Geometry check sheet. Reference: the model listing, model coordinates, mm. Face numbers are marked on the shaded views. A direction names the side the tool comes from. Give positions to 0.01 mm unless a question says otherwise; leave off trailing zeros. Order: outer loops, then holes, each group sorted by start corner. A loop starts at its lowest first (then second) coordinate and runs counter-clockwise, first axis right, second up. Notation, with made-up numbers: M -12,57.25 L 20,57.25 A37 ccw 20,94.25 Z; hole C -34.5,-9 d4. An arc over 180 degrees is marked long. Answer as a JSON object with one key per item and string values. Group by question number.
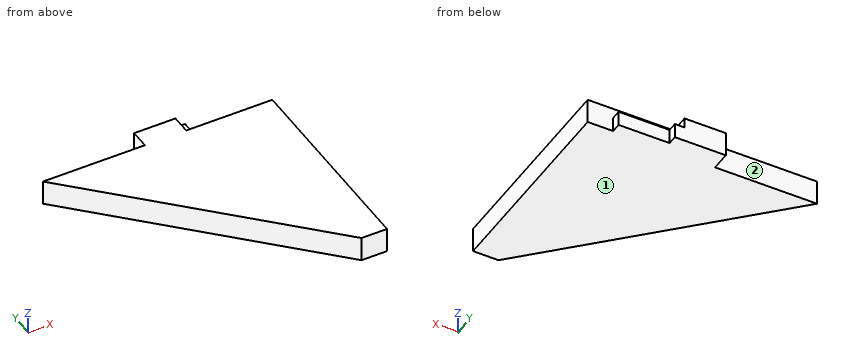
from build123d import *

# Parameters (mm, degrees)
F0_W     = 10.287
F0_H     = 4.745708
F0_W_2   = 6.35
F0_H_2   = 50.8
F1_DEPTH = 6.223
F0_W_3   = 12.7
F0_H_3   = 2.413
F2_DEPTH = 3.683


with BuildPart() as f1:
    # F0 (on Top) → F1 (new body)
    with BuildSketch(Plane.XY):
        Polygon((-25.4, 25.4), (25.4, -25.4), (25.4, 25.4), (12.7, 25.4), (10.287, 25.4), (0, 25.4), align=None)
        with Locations((5.1435, 27.772854)):
            Rectangle(F0_W, F0_H)
        with Locations((28.575, 0)):
            Rectangle(F0_W_2, F0_H_2)
    extrude(amount=F1_DEPTH)

    # F0 (on Top) → F2 (join)
    with BuildSketch(Plane.XY):
        Polygon((10.287, 25.4), (12.7, 25.4), (12.7, 27.813), (12.7, 30.145708), (10.287, 30.145708), align=None)
        with Locations((19.05, 26.6065)):
            Rectangle(F0_W_3, F0_H_3)
    extrude(amount=F2_DEPTH)


solid = f1.part
1. Cross-section at D-D (x = 28.5). Record the cut outline in (y, z).
2. Access from +Z, -Z, +X, -X, +Y, -Y to the whole of each face (thin tool, end or side, straight path). Record for the marked faces 1 and 2.
3. Cross-section at A-A (z = 5.25). Record the cut outline in (x, y).
4. Cross-section at B-B (x = 21). Record the cut outline in (y, z).
5. Thickness scan on line 1 along X through (y, z) = (28.5, 2.25); line 2 along Y through (x, z) = (28.5, 3); line 3 along Y through (x, z) = (23, 1). Record the ranges inside material, lowest first. Write a range as [from, to].
6. Depth check by flat-ended pin: pin 1 (3 mm diameter, centred on y = 27, z = 5.5, fed in from +X); pin 2 (1 mm diameter, centred on x = 14, z = 3.5, fed in from -Y); pin 3 (1.2 mm diameter, centred on y = 29, z = 2, fed in from +X). Enter the tip coordinate at first touch or a pass-through.
7. Cross-section at C-C (y = 6). Record the cut outline in (x, z).
Report:
{
 "1": {"outline": "M -25.4,0 L 25.4,0 L 25.4,6.22 L -25.4,6.22 Z"},
 "2": {"face 1": "-Z, +X, -X, +Y, -Y", "face 2": "+Z, -Z, -X, +Y"},
 "3": {"outline": "M -25.4,25.4 L 25.4,-25.4 L 31.75,-25.4 L 31.75,25.4 L 10.29,25.4 L 10.29,30.15 L 0,30.15 L 0,25.4 Z"},
 "4": {"outline": "M -21,0 L 27.81,0 L 27.81,3.68 L 25.4,3.68 L 25.4,6.22 L -21,6.22 Z"},
 "5": {"line 1": "x = [0, 12.7]", "line 2": "y = [-25.4, 25.4]", "line 3": "y = [-23, 27.81]"},
 "6": {"pin 1": "stops at x = 10.29", "pin 2": "stops at y = -14.5", "pin 3": "stops at x = 12.7"},
 "7": {"outline": "M -6,0 L 31.75,0 L 31.75,6.22 L -6,6.22 Z"}
}
